Can you work these out from the model? Positions are in its coordinate system, mm. Face numbers are marked on the shaded views. Round coordinates to 2 decimals unless told otherwise and drop trailing zeros. Write item = value, one per line.
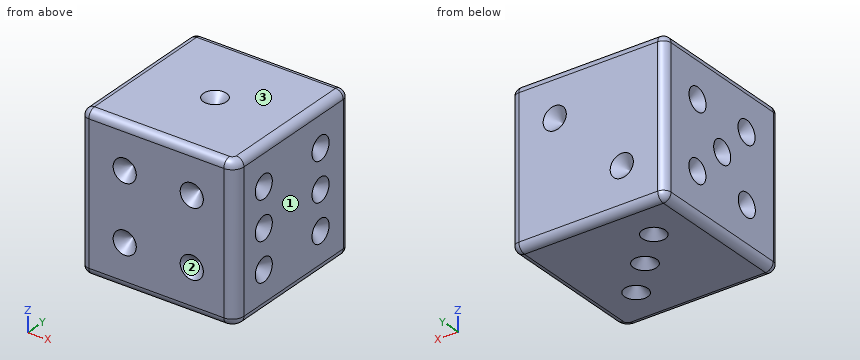
from build123d import *

# Parameters (mm, degrees)
F0_W         = 20
F0_H         = 20
F1_DEPTH     = 20
F2_R         = 1.5
F3_DEPTH     = 1.5
F4_R         = 1.5
F5_DEPTH     = 1.5
F6_R         = 1
F7_SIZE      = 1.49999
F8_R         = 1.5
F9_DEPTH     = 1.5
F10_SIZE     = 1.49999
F11_SIZE     = 1.49999
F12_T1_DEPTH = 20
F12_T4_ANGLE = 90
F12_T6_ANGLE = 90
F13_SIZE     = 1.49999
F14_R        = 1.5
F15_DEPTH    = 1.5
F16_SIZE     = 1.49999
F17_R        = 1.5
F18_DEPTH    = 1.5
F19_SIZE     = 1.49999
F20_R        = 1.5
F21_DEPTH    = 1.5
F22_SIZE     = 1.49999


# Not quite as in the source:
# - a fillet or chamfer that OpenCascade refuses, or shapes differently, is made with other operations: its cross-section is extruded or revolved along the edge and cut away or added
# - a fillet or chamfer is up to 0.001 mm smaller than in the source, because OpenCascade refuses the exact size


with BuildPart() as f1:
    # F0 (on Top) → F1 (new body)
    with BuildSketch(Plane.XY):
        with Locations((10, 10)):
            Rectangle(F0_W, F0_H)
    extrude(amount=F1_DEPTH)

    # F2 (on face) → F3 (cut)
    with BuildSketch(Plane.XY.offset(20)):
        with Locations((10, 10)):
            Circle(F2_R)
    extrude(amount=-F3_DEPTH, mode=Mode.SUBTRACT)

    # F4 (on face) → F5 (cut)
    with BuildSketch(Plane(origin=(0, 20, 0), x_dir=(-1, 0, 0), z_dir=(0, 1, 0))):
        with Locations((-14.3431457505, 14.3431457505)):
            Circle(F4_R)
        with Locations((-5.6568542495, 5.6568542495)):
            Circle(F4_R)
    extrude(amount=-F5_DEPTH, mode=Mode.SUBTRACT)

    # F6
    f6_edges = [f1.edges().sort_by_distance(p)[0] for p in [
        (0, 0, 10),
        (0, 10, 0),
        (20, 20, 10),
        (0, 20, 10),
        (10, 20, 20),
        (0, 10, 20),
        (10, 0, 0),
        (20, 10, 0),
        (20, 10, 20),
        (10, 0, 20),
        (10, 20, 0),
    ]]
    fillet(f6_edges, radius=F6_R)

    # F7 (size 1.5 in the source; OpenCascade refuses exactly that, so slightly less here)
    f7_edges = [f1.edges().sort_by_distance(p)[0] for p in [
        (7.156854, 18.5, 5.656854),
    ]]
    chamfer(f7_edges, length=F7_SIZE)

    # F8 (on face) → F9 (cut)
    with BuildSketch(Plane(origin=(0, 0, 0), x_dir=(1, 0, 0), z_dir=(0, 0, -1))):
        with Locations((5.6568542495, -14.3431457505)):
            Circle(F8_R)
        with Locations((10, -10)):
            Circle(F8_R)
        with Locations((14.3431457505, -5.6568542495)):
            Circle(F8_R)
    extrude(amount=-F9_DEPTH, mode=Mode.SUBTRACT)

    # F10 (size 1.5 in the source; OpenCascade refuses exactly that, so slightly less here)
    f10_edges = [f1.edges().sort_by_distance(p)[0] for p in [
        (15.843146, 18.5, 14.343146),
    ]]
    chamfer(f10_edges, length=F10_SIZE)

    # F11 (size 1.5 in the source; OpenCascade refuses exactly that, so slightly less here)
    f11_edges = [f1.edges().sort_by_distance(p)[0] for p in [
        (8.5, 10, 18.5),
    ]]
    chamfer(f11_edges, length=F11_SIZE)

    # F12: fillet of radius 1.5 on 1 edges, made by hand

    # F12_s2 → F12_t1 (cut)
    with BuildSketch(Plane.XY):
        with BuildLine():
            ThreePointArc((20, 1.5), (19.5606601718, 0.4393398282), (18.5, 0))
            Line((18.5, 0), (20, 0))
            Line((20, 0), (20, 1.5))
        make_face()
    extrude(amount=F12_T1_DEPTH, mode=Mode.SUBTRACT)

    # F12_s3 → F12_t4 (revolve, cut)
    with BuildSketch(Plane.XZ.offset(-1.5)):
        with BuildLine():
            ThreePointArc((19, 0), (19.7071067812, 0.2928932188), (20, 1))
            Line((20, 1), (20, 0))
            Line((20, 0), (19, 0))
        make_face()
    revolve(axis=Axis((18.5, 1.5, 0), (0, 0, -1)), revolution_arc=F12_T4_ANGLE, mode=Mode.SUBTRACT)

    # F12_s5 → F12_t6 (revolve, cut)
    with BuildSketch(Plane.YZ.offset(18.5)):
        with BuildLine():
            ThreePointArc((1, 20), (0.2928932188, 19.7071067812), (0, 19))
            Line((0, 19), (0, 20))
            Line((0, 20), (1, 20))
        make_face()
    revolve(axis=Axis((18.5, 1.5, 20), (0, 0, 1)), revolution_arc=F12_T6_ANGLE, mode=Mode.SUBTRACT)

    # F13 (size 1.5 in the source; OpenCascade refuses exactly that, so slightly less here)
    f13_edges = [f1.edges().sort_by_distance(p)[0] for p in [
        (4.156854, 14.343146, 1.5),
        (8.5, 10, 1.5),
        (12.843146, 5.656854, 1.5),
    ]]
    chamfer(f13_edges, length=F13_SIZE)

    # F14 (on face) → F15 (cut)
    with BuildSketch(Plane.XZ):
        with Locations((5.6568542495, 5.6568542495)):
            Circle(F14_R)
        with Locations((5.6568542495, 14.3431457505)):
            Circle(F14_R)
        with Locations((14.3431457505, 14.3431457505)):
            Circle(F14_R)
        with Locations((14.3431457505, 5.6568542495)):
            Circle(F14_R)
    extrude(amount=-F15_DEPTH, mode=Mode.SUBTRACT)

    # F16 (size 1.5 in the source; OpenCascade refuses exactly that, so slightly less here)
    f16_edges = [f1.edges().sort_by_distance(p)[0] for p in [
        (4.156854, 1.5, 14.343146),
        (12.843146, 1.5, 14.343146),
        (4.156854, 1.5, 5.656854),
        (12.843146, 1.5, 5.656854),
    ]]
    chamfer(f16_edges, length=F16_SIZE)

    # F17 (on face) → F18 (cut)
    with BuildSketch(Plane(origin=(0, 0, 0), x_dir=(0, -1, 0), z_dir=(-1, 0, 0))):
        with Locations((-14.3431457505, 14.3431457505)):
            Circle(F17_R)
        with Locations((-5.7128249468, 14.3996758016)):
            Circle(F17_R)
        with Locations((-10, 10)):
            Circle(F17_R)
        with Locations((-14.3682878079, 5.6818850556)):
            Circle(F17_R)
        with Locations((-5.6568542495, 5.6568542495)):
            Circle(F17_R)
    extrude(amount=-F18_DEPTH, mode=Mode.SUBTRACT)

    # F19 (size 1.5 in the source; OpenCascade refuses exactly that, so slightly less here)
    f19_edges = [f1.edges().sort_by_distance(p)[0] for p in [
        (1.5, 15.843146, 14.343146),
        (1.5, 15.868288, 5.681885),
        (1.5, 11.5, 10),
        (1.5, 7.212825, 14.399676),
        (1.5, 7.156854, 5.656854),
    ]]
    chamfer(f19_edges, length=F19_SIZE)

    # F20 (on face) → F21 (cut)
    with BuildSketch(Plane.YZ.offset(20)):
        with Locations((15, 15)):
            Circle(F20_R)
        with Locations((5, 15)):
            Circle(F20_R)
        with Locations((5, 10)):
            Circle(F20_R)
        with Locations((15, 10)):
            Circle(F20_R)
        with Locations((15, 5)):
            Circle(F20_R)
        with Locations((5, 5)):
            Circle(F20_R)
    extrude(amount=-F21_DEPTH, mode=Mode.SUBTRACT)

    # F22 (size 1.5 in the source; OpenCascade refuses exactly that, so slightly less here)
    f22_edges = [f1.edges().sort_by_distance(p)[0] for p in [
        (18.5, 13.5, 5),
        (18.5, 13.5, 10),
        (18.5, 3.5, 10),
        (18.5, 3.5, 5),
        (18.5, 3.5, 15),
        (18.5, 13.5, 15),
    ]]
    chamfer(f22_edges, length=F22_SIZE)


solid = f1.part
1. I need wall thicknesses on line 1 (X direction, y = 4, z = 6); line 2 (X direction, y = 19.25, z = 13.25); line 3 (Y direction, x = 6.25, z = 13.75). Which ranges of each line are inside material? Lowest first, please. Write a range as [from, to].
Entries:
line_1 = [0, 19.91]
line_2 = [0.03, 19.97]
line_3 = [0.66, 20]
2. I'm going to push a flat-ended pin straight in: pin 1 (2.5 mm diameter, centred on x = 5.66, z = 5.66, fed in from -Y). Where does the tip first touch, or does it pass through?
Entries:
pin_1 = 0.25
3. We'd pull the mould along Z, two halves only. Please class the marked faces 1, 2 and 3: released by +Z, released by -Z, zero draft, split by the parting line, or undercut.
Entries:
face_1 = zero draft
face_2 = undercut
face_3 = released by +Z
